```python
from build123d import *

# Parameters (mm, degrees)
SKETCH1_R           = 22.86
BOSS_EXTRUDE1_DEPTH = 22.86
SKETCH3_R           = 15.24
BOSS_EXTRUDE2_DEPTH = 55.88
SKETCH4_R           = 22.86
BOSS_EXTRUDE3_DEPTH = 22.86
FILLET3_R           = 2.54
SKETCH5_R           = 2.5
CUT_EXTRUDE1_DEPTH  = 7
FILLET4_R           = 1.27
SKETCH8_R           = 3.175
BOSS_EXTRUDE4_DEPTH = 12.7


with BuildPart() as part:
    # Sketch1 → Boss-Extrude1 (new body)
    with BuildSketch(Plane(origin=(0, 0, 0), x_dir=(1, 0, 0), z_dir=(0, 1, 0))):
        Circle(SKETCH1_R)
    extrude(amount=BOSS_EXTRUDE1_DEPTH)

    # Sketch3 → Boss-Extrude2 (add)
    with BuildSketch(Plane(origin=(0, 22.86, 0), x_dir=(1, 0, 0), z_dir=(0, 1, 0))):
        Circle(SKETCH3_R)
    extrude(amount=BOSS_EXTRUDE2_DEPTH)

    # Sketch4 → Boss-Extrude3 (add)
    with BuildSketch(Plane(origin=(0, 78.74, 0), x_dir=(1, 0, 0), z_dir=(0, 1, 0))):
        Circle(SKETCH4_R)
    extrude(amount=BOSS_EXTRUDE3_DEPTH)

    # Fillet3
    fillet3_edges = [part.edges().sort_by_distance(p)[0] for p in [
        (-22.86, 101.6, 0),
        (-22.86, 0, 0),
    ]]
    fillet(fillet3_edges, radius=FILLET3_R)

    # Sketch5 → Cut-Extrude1 (cut)
    with BuildSketch(Plane(origin=(0, 101.6, 0), x_dir=(1, 0, 0), z_dir=(0, 1, 0))):
        Circle(SKETCH5_R)
    extrude(amount=-CUT_EXTRUDE1_DEPTH, mode=Mode.SUBTRACT)

    # Fillet4
    fillet4_edges = [part.edges().sort_by_distance(p)[0] for p in [
        (-2.5, 101.6, 0),
    ]]
    fillet(fillet4_edges, radius=FILLET4_R)

    # Sketch8 → Boss-Extrude4 (add)
    with BuildSketch(Plane.XZ):
        Circle(SKETCH8_R)
    extrude(amount=BOSS_EXTRUDE4_DEPTH)


solid = part.part
```
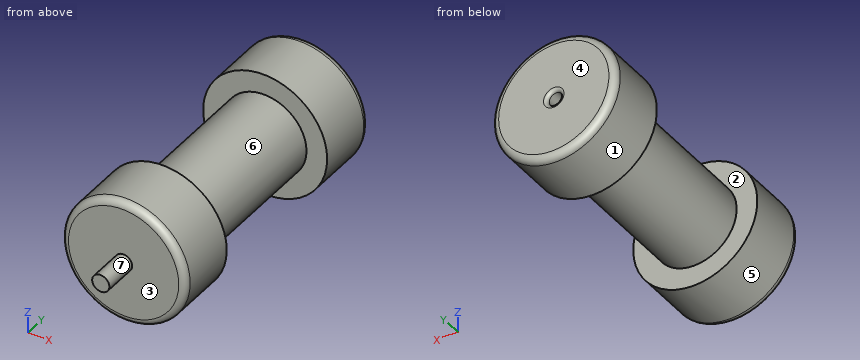
Input: part model. Units: mm. Frame: model coordinates. Face numbers are marked on the shaded views. A direction names the side the tool comes from. Coordinates: 2 decimals unless noted, no trailing zeros. Write each loop counter-clockwise with the first axis right and the second up, starting at its lowest first coordinate (ties: lowest second). Pieces come first, ordered by that corner, then holes. Notation, with made-up numbers: (48, 74.5) - (77, 74.5) arc R22 cw to (77, 107.5) - close; hole circle Ø3 at (58.25, 38.25). An arc over 180 degrees is marked (long way). Put each result on its own line as item: value. Start each with the question number.
1) Cut plane B-B (x = 0). Return the cut outline in (y, z) (3 decimals).
2) Cut plane D-D (y = 6). Return the cut outline in (x, z), plus the area to 3 significant figures.
3) Cut plane C-C (y = 51.5). Return the cut outline in (x, z).
4) Ray query, L1, parallel to X at y = 96.4, z = 0; L2, parallel to Y at x = 7, z = 18. Return the intervals inside material, ascending.
5) Contact query for flat-ended pins moving along their axis: pin 1 (10 mm diameter, centred on x = -1, z = -11, fed in from -Y); pin 2 (6.5 mm diameter, centred on x = 0, z = 0, fed in from +Y); pin 3 (13.5 mm diameter, centred on x = 3, z = -2, fed in from -Y); pin 4 (8 mm diameter, centred on x = 10.5, y = 62, fed in from -Z). Output: stop coordinate, or through.
6) Mould query, pull axis Y, two halves, no side actions, for the marked faces 1, 2, 3 and 4. Classes: pulls with the +Y half, pulls with the -Y half, needs draft (parallel to the pull), parting line crosses it, or undercut.
7) Reachability of the marked faces 5, 6 and 7 from +Z, -Z, +X, -X, +Y, -Y: full face, straight path, thin tool, end or side. Return the list, or none.
8) Cut plane A-A (z = 0). Return the cut outline in (x, y) (3 decimals), plus the area to 3 significant figures.
Resolved:
1. outline: (-12.7, -3.175) - (0, -3.175) - (0, -20.32) arc R2.54 ccw to (2.54, -22.86) - (22.86, -22.86) - (22.86, -15.24) - (78.74, -15.24) - (78.74, -22.86) - (99.06, -22.86) arc R2.54 ccw to (101.6, -20.32) - (101.6, -3.77) arc R1.27 ccw to (100.33, -2.5) - (94.6, -2.5) - (94.6, 2.5) - (100.33, 2.5) arc R1.27 ccw to (101.6, 3.77) - (101.6, 20.32) arc R2.54 ccw to (99.06, 22.86) - (78.74, 22.86) - (78.74, 15.24) - (22.86, 15.24) - (22.86, 22.86) - (2.54, 22.86) arc R2.54 ccw to (0, 20.32) - (0, 3.175) - (-12.7, 3.175) - close
2. outline: circle Ø45.72 at (0, 0)
2. area: 1,640 mm2
3. outline: circle Ø30.48 at (0, 0)
4. L1: x = -22.86 to -2.5, 2.5 to 22.86
4. L2: y = 0 to 22.86, 78.74 to 101.6
5. pin 1: stops at y = 0
5. pin 2: stops at y = 101.49
5. pin 3: stops at y = -12.7
5. pin 4: stops at z = -13.78
6. face 1: needs draft
6. face 2: undercut
6. face 3: pulls with the -Y half
6. face 4: pulls with the +Y half
7. face 5: +Y, -Y
7. face 6: none
7. face 7: -Y
8. outline: (-22.86, 2.54) arc R2.54 ccw to (-20.32, 0) - (-3.175, 0) - (-3.175, -12.7) - (3.175, -12.7) - (3.175, 0) - (20.32, 0) arc R2.54 ccw to (22.86, 2.54) - (22.86, 22.86) - (15.24, 22.86) - (15.24, 78.74) - (22.86, 78.74) - (22.86, 99.06) arc R2.54 ccw to (20.32, 101.6) - (3.77, 101.6) arc R1.27 ccw to (2.5, 100.33) - (2.5, 94.6) - (-2.5, 94.6) - (-2.5, 100.33) arc R1.27 ccw to (-3.77, 101.6) - (-20.32, 101.6) arc R2.54 ccw to (-22.86, 99.06) - (-22.86, 78.74) - (-15.24, 78.74) - (-15.24, 22.86) - (-22.86, 22.86) - close
8. area: 3,830 mm2
